Can you work these out from the model? Positions are in its coordinate system, mm. A direction names the side the tool comes from. Give positions to 0.01 mm unless a question says otherwise; leave off trailing zeros. Loops run counter-clockwise (first coordinate to the right, second up) from the corner with the lowest first, then second, coordinate; pieces in that order, holes last. Notation, with made-up numbers: (14, 55) - (34, 55) arc R19 ccw to (34, 76) - close; hole circle Ø3 at (0, 17). An arc over 180 degrees is marked (long way). Answer as a JSON object with one key per item and string values. Group by question number.
Item 1: Suppose I cut it at A-A on z = -206.5. Write out the boundary of the cut face in (x, y).
Item 2: Please list where these lines run through material, in increasing order: L1, parallel to X at y = -14, z = -232; L2, parallel to X at y = 14, z = -126; L3, parallel to Y at x = 14, z = -219.5.
Item 3: Which directions (+Z, -Z, +X, -X, +Y, -Y) give clear straight access to the entire face, cutting with the end or side of a thin tool? Please do faces 1 (the flat face through (8.6, -15.462, 4.2)), 2 (the flat face through (-11.725, 12, 4)).
Item 4: Suppose I cut it at C-C on x = -6. Write out the boundary of the cut face in (y, z), and give its area (3 significant figures).
Item 5: Suppose I cut it at B-B on y = 1. Write out the boundary of the cut face in (x, z), and give its area (3 significant figures).
Item 6: Will these pins go through, and if not, where does the flat tip stop? pin 1 (9 mm diameter, centred on x = 8.27, z = 0, fed in from +Y); pin 2 (7 mm diameter, centred on x = 8.27, z = 232.01, fed in from +Y); pin 3 (8 mm diameter, centred on y = 12.5, z = 77.5, fed in from +X).
from build123d import *

# Parameters (mm, degrees)
BOSS_EXTRUDE1_DEPTH = 302.01
SKETCH2_R           = 4
CUT_EXTRUDE1_DEPTH  = 20
CUT_EXTRUDE2_DEPTH  = 8
LPATTERN1_COUNT     = 3
LPATTERN1_PITCH     = 232.01


with BuildPart() as part:
    # Sketch1 → Boss-Extrude1 (new, symmetric)
    with BuildSketch(Plane.XY):
        Polygon((-16.725146199, 34.538011696), (-11.725146199, 34.538011696), (-11.725146199, -10.461988304), (33.274853801, -10.461988304), (33.274853801, -15.461988304), (-16.725146199, -15.461988304), align=None)
    extrude(amount=BOSS_EXTRUDE1_DEPTH, both=True)

    # Sketch2 → Cut-Extrude1 (cut)
    with BuildSketch(Plane(origin=(0, -10.461988304, 0), x_dir=(1, 0, 0), z_dir=(0, 1, 0))):
        with Locations(Location((8.274853801, 232.01, 0), (0, 0, 270))):
            Circle(SKETCH2_R)
    cut_extrude1 = extrude(amount=-CUT_EXTRUDE1_DEPTH, mode=Mode.SUBTRACT)

    # Sketch3 → Cut-Extrude2 (cut)
    with BuildSketch(Plane(origin=(0, -10.461988304, 0), x_dir=(1, 0, 0), z_dir=(0, 1, 0))):
        Polygon((33.274853801, 255.912277714), (3.274853801, 302.01), (33.274853801, 302.01), align=None)
    cut_extrude2 = extrude(amount=-CUT_EXTRUDE2_DEPTH, mode=Mode.SUBTRACT)

    # Mirror2: Cut-Extrude2 across plane
    add(cut_extrude2.mirror(Plane.XY), mode=Mode.SUBTRACT)

    # LPattern1: Cut-Extrude1 ×3
    with Locations(*[(0, 0, i * LPATTERN1_PITCH) for i in range(1, LPATTERN1_COUNT)]):
        add(cut_extrude1, mode=Mode.SUBTRACT)


solid = part.part
Worked out:
{
 "1": {"outline": "(-16.73, -15.46) - (33.27, -15.46) - (33.27, -10.46) - (-11.73, -10.46) - (-11.73, 34.54) - (-16.73, 34.54) - close"},
 "2": {"L1": "x = -16.73 to 4.27, 12.27 to 33.27", "L2": "x = -16.73 to -11.73", "L3": "y = -15.46 to -10.46"},
 "3": {"face 1": "+Z, -Z, +X, -X, -Y", "face 2": "+Z, -Z, +X, +Y"},
 "4": {"outline": "(-15.46, -302.01) - (-10.46, -302.01) - (-10.46, 302.01) - (-15.46, 302.01) - close", "area": "3,020 mm2"},
 "5": {"outline": "(-16.73, -302.01) - (-11.73, -302.01) - (-11.73, 302.01) - (-16.73, 302.01) - close", "area": "3,020 mm2"},
 "6": {"pin 1": "stops at y = -10.46", "pin 2": "passes through", "pin 3": "stops at x = -11.73"}
}
